Check sheet for the modelled part. Datum: model origin and axes. Units: mm. Face numbers are marked on the shaded views. A direction names the side the tool comes from. Give positions to 0.01 mm unless a question says otherwise; leave off trailing zeros. Loops run counter-clockwise (first coordinate to the right, second up) from the corner with the lowest first, then second, coordinate; pieces in that order, holes last. Notation, with made-up numbers: (1.5, -36.5) -> (46.5, -36.5) arc R26 cw to (46.5, -22.5) -> close; hole circle Ø3 at (-11, 53). An arc over 180 degrees is marked (long way). Write each question's results on one line, items separated by ' | '. Start each with the question number.
1. Cross-section at C-C on z = 0.5. Record the boundary of the cut face in (x, y).
2. Cross-section at A-A on x = 0. Record the boundary of the cut face in (y, z), and give its area (3 significant figures).
3. Mould release check, pull along X, two halves, no side actions. Record for the marked faces 1, 2 and 3: +X half, -X half, draft (parallel to the pull), parting line (faces both ways), or undercut.
4. Tool access check on the marked faces 4 and 5. Record the directions out of +Z, -Z, +X, -X, +Y, -Y that give a thin tool (end or side, any length) a straight path to the whole face; none if there is none.
5. Material ranges on L1, parallel to Y at x = 0, z = -5.2; L2, parallel to Y at x = 3, z = 0.25; L3, parallel to Y at x = 3.5, z = 2.75, recorded low to high. Write a range as from..to.
6. Gauge pin test, flat ends, axial feed: pin 1 Ø3 at (y, z) = (1, -3) entering from -X; pin 2 Ø1 at (x, z) = (-1, -0.5) entering from +Y; pin 3 Ø4 at (x, z) = (0, -3) entering from -Y. Record the tip position at first contact, or that the pin passes through.
Autodesk Fusion 360 part; units mm, degrees
sketch "Sketch1" plane through (0, 0, 0) normal (0, 0, 1) x (1, 0, 0)
  circle A0 centre (0, 0) radius 4.3
  circle A1 centre (0, 0) radius 3.95
  circle A2 centre (0, 0) radius 2.5
  circle A3 centre (0, 0) radius 3.3
  circle A4 centre (0, 0) radius 2.843
  circle A5 centre (0, 0) radius 2.75
  dimension "d1" = 8.6
  dimension "d2" = 7.9
  dimension "d3" = 5
  dimension "d4" = 6.6
  dimension "d14" = 5.5
extrude "Extrude3" add sketch "Sketch1" against normal blind 7 contours A1 | A3 | A4 | A5
extrude "Extrude4" add sketch "Sketch1" along normal blind 3 contours A0 | A1
extrude "Extrude5" add sketch "Sketch1" against normal blind 0.5 contours A3 | A4
extrude "Extrude7" cut 1 faces at (3.0117, -0.2881, 0) along direction (0, 0, -1) blind 3
extrude "Extrude8" cut 1 faces at (4.1673, -0.2136, 0) along direction (0, 0, 1) blind 2
chamfer "Chamfer1" distance 1 distance2 3 1 edges at (-3.6827, 1.4284, -7) measured on face at (3.4427, -0.3204, -7)
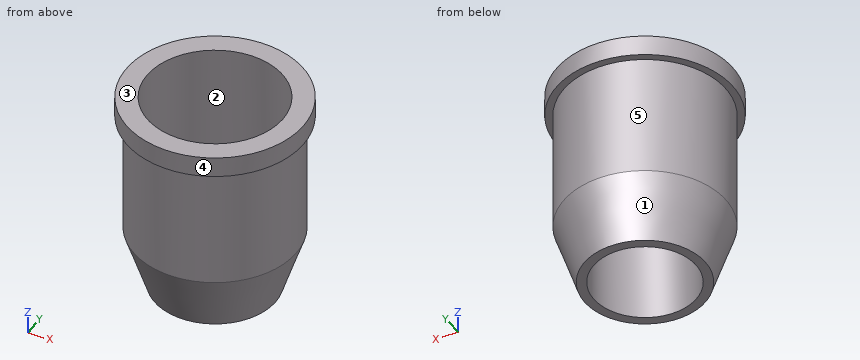
Geometry says:
1) outline: circle Ø7.9 at (0, 0); hole circle Ø6.6 at (0, 0)
2) outline: (-4.3, 2) -> (-3.95, 2) -> (-3.95, -4) -> (-2.95, -7) -> (-2.5, -7) -> (-2.5, -3) -> (-3.3, -3) -> (-3.3, 3) -> (-4.3, 3) -> close; (2.5, -7) -> (2.95, -7) -> (3.95, -4) -> (3.95, 2) -> (4.3, 2) -> (4.3, 3) -> (3.3, 3) -> (3.3, -3) -> (2.5, -3) -> close | area: 17.1 mm^2
3) face 1: parting line | face 2: undercut | face 3: draft
4) face 4: +Z, -Z | face 5: -Z
5) L1: -3.55..-2.5, 2.5..3.55 | L2: -2.57..-1.37, 1.37..2.57 | L3: -2.5..2.5
6) pin 1: x = -3.95 | pin 2: y = 3.92 | pin 3: y = -3.95
